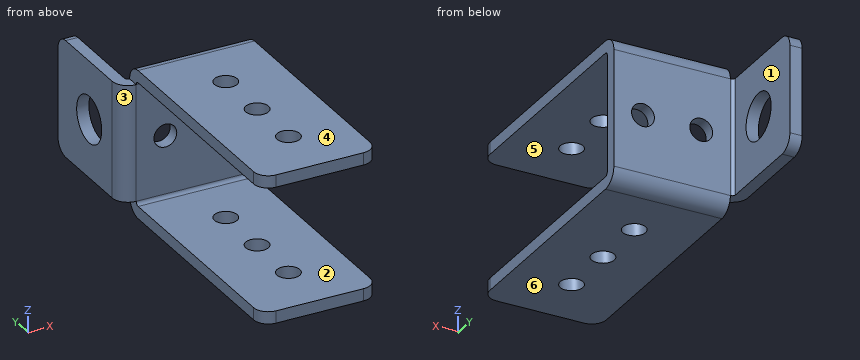
```python
from build123d import *

# Parameters (mm, degrees)
BASE_FLANGE1_START = -12.7
BASE_FLANGE1_DEPTH = 25.4
EDGE_FLANGE1_DEPTH = 25.4
SKETCH9_R          = 5.08
CUT_EXTRUDE1_DEPTH = 86.828419099
SKETCH10_R         = 2.4892
CUT_EXTRUDE2_DEPTH = 85.303992818
CUT_EXTRUDE3_REACH = 65.202
SKETCH11_R         = 2.4892
FILLET1_R          = 3.175


# Read off the part's stored shape, not the designer's step: Base-Flange1
# Sheet-metal steps are written as plain solids
with BuildPart() as part:
    # Base-Flange1 outline → Base-Flange1 (new body)
    with BuildSketch(Plane(origin=(0, 0, 0), x_dir=(0, 0, -1), z_dir=(1, 0, 0)).offset(BASE_FLANGE1_START)):
        with BuildLine():
            Line((26.924, 50.038), (26.924, 0))
            Line((26.924, 0), (29.591, 0))
            Line((29.591, 0), (29.591, 50.038))
            ThreePointArc((29.591, 50.038), (28.586669153, 52.462669153), (26.162, 53.467))
            Line((26.162, 53.467), (0.762, 53.467))
            ThreePointArc((0.762, 53.467), (-1.662669153, 52.462669153), (-2.667, 50.038))
            Line((-2.667, 50.038), (-2.667, 0))
            Line((-2.667, 0), (0, 0))
            Line((0, 0), (0, 50.038))
            ThreePointArc((0, 50.038), (0.223184633, 50.576815367), (0.762, 50.8))
            Line((0.762, 50.8), (26.162, 50.8))
            ThreePointArc((26.162, 50.8), (26.700815367, 50.576815367), (26.924, 50.038))
        make_face()
    extrude(amount=BASE_FLANGE1_DEPTH)

    # Edge-Flange1 section (across the edge) → Edge-Flange1 (add)
    with BuildSketch(Plane(origin=(-13.462, 53.467, -26.162), x_dir=(1, 0, 0), z_dir=(0, 0, 1))):
        with BuildLine():
            Line((-2.667, 0.762), (-2.667, 22.733))
            Line((-2.667, 22.733), (0, 22.733))
            Line((0, 22.733), (0, 0.762))
            ThreePointArc((0, 0.762), (0.223184633, 0.223184633), (0.762, 0))
            Line((0.762, 0), (0.762, -2.667))
            ThreePointArc((0.762, -2.667), (-1.662669153, -1.662669153), (-2.667, 0.762))
        make_face()
    extrude(amount=EDGE_FLANGE1_DEPTH)

    # Sketch9 → Cut-Extrude1 (cut, through all)
    with BuildSketch(Plane(origin=(-13.462, 0, 0), x_dir=(0, 0, -1), z_dir=(1, 0, 0))):
        with Locations(Location((13.462, 63.5, 0), (0, 0, 90))):
            Circle(SKETCH9_R)
    extrude(amount=-CUT_EXTRUDE1_DEPTH, mode=Mode.SUBTRACT)

    # Sketch10 → Cut-Extrude2 (cut, through all)
    with BuildSketch(Plane.XY.offset(2.667)):
        with Locations((0, 12.7)):
            Circle(SKETCH10_R)
        with Locations((0, 25.4)):
            Circle(SKETCH10_R)
        with Locations((0, 38.1)):
            Circle(SKETCH10_R)
    extrude(amount=-CUT_EXTRUDE2_DEPTH, mode=Mode.SUBTRACT)

    # Sketch11 → Cut-Extrude3 (cut, up to next)
    with BuildSketch(Plane(origin=(0, 53.467, 0), x_dir=(1, 0, 0), z_dir=(0, 1, 0)), mode=Mode.PRIVATE) as cut_extrude3_sk1:
        with Locations(Location((-6.35, 13.462, 0), (0, 0, 270))):
            Circle(SKETCH11_R)
    cut_extrude3_tool1 = extrude(cut_extrude3_sk1.sketch, amount=-CUT_EXTRUDE3_REACH, mode=Mode.PRIVATE) & part.part
    # Sketch11 → Cut-Extrude3 (cut, up to next)
    with BuildSketch(Plane(origin=(0, 53.467, 0), x_dir=(1, 0, 0), z_dir=(0, 1, 0)), mode=Mode.PRIVATE) as cut_extrude3_sk2:
        with Locations(Location((6.35, 13.462, 0), (0, 0, 270))):
            Circle(SKETCH11_R)
    cut_extrude3_tool2 = extrude(cut_extrude3_sk2.sketch, amount=-CUT_EXTRUDE3_REACH, mode=Mode.PRIVATE) & part.part
    add(cut_extrude3_tool1.solids().sort_by_distance((-6.35, 53.467, -13.462))[0], mode=Mode.SUBTRACT)
    add(cut_extrude3_tool2.solids().sort_by_distance((6.35, 53.467, -13.462))[0], mode=Mode.SUBTRACT)

    # Fillet1
    fillet1_edges = [part.edges().sort_by_distance(p)[0] for p in [
        (-12.7, 0, 1.3335),
        (-12.7, 0, -28.2575),
        (12.7, 0, 1.3335),
        (-14.7955, 76.2, -26.162),
        (-14.7955, 76.2, -0.762),
        (12.7, 0, -28.2575),
    ]]
    fillet(fillet1_edges, radius=FILLET1_R)


solid = part.part
```
Input: part model. Units: mm. Frame: model coordinates. Face numbers are marked on the shaded views. A direction names the side the tool comes from. Round coordinates to 2 decimals unless told otherwise and drop trailing zeros. Loops run counter-clockwise (first coordinate to the right, second up) from the corner with the lowest first, then second, coordinate; pieces in that order, holes last. Notation, with made-up numbers: (89.25, 45) -> (143.25, 45) arc R18 ccw to (143.25, 61) -> close; hole circle Ø6 at (58, 84). An arc over 180 degrees is marked (long way). Write each question's results on one line, items separated by ' | '.
1. Ray query, line 1 (Z direction, x = -15.55, y = 63.5); line 2 (Z direction, x = -10.25, y = 17.5); line 3 (Y direction, x = 0, z = 1.6). Return the intervals inside material, ascending. Write a range as from..to.
Geometry results:
line 1: -26.16..-18.54, -8.38..-0.76 | line 2: -29.59..-26.92, 0..2.67 | line 3: 0..10.21, 15.19..22.91, 27.89..35.61, 40.59..52.52
2. Section B-B (y = 25.4). Return loops of the section in (x, z), and give its area (3 significant figures).
Geometry results:
outline: (-12.7, -29.59) -> (-2.49, -29.59) -> (-2.49, -26.92) -> (-12.7, -26.92) -> close; (-12.7, 0) -> (-2.49, 0) -> (-2.49, 2.67) -> (-12.7, 2.67) -> close; (2.49, -29.59) -> (12.7, -29.59) -> (12.7, -26.92) -> (2.49, -26.92) -> close; (2.49, 0) -> (12.7, 0) -> (12.7, 2.67) -> (2.49, 2.67) -> close | area: 109 mm2
3. Set-up query: the marked faces 1, 2 and 3. Return all of +Z, -Z, +X, -X, +Y, -Y with unobstructed straight access to the full face (end or side cutting, diameter ignored); none if empty.
Geometry results:
face 1: +Z, -Z, +X, +Y | face 2: +X, -X, -Y | face 3: +Z, -Z, -X, -Y
4. First-contact query: P1, Ø4.5, axis at x = 0, y = 38.1, coming from the -Z side; P2, Ø6.5, axis at x = -6.35, z = -13.462, coming from the -Y side; P3, Ø2, axis at x = 9.5, z = -4, coming from the +Y side; P4, Ø1.5, axis at y = 51.5, z = -5.5, coming from the -X side. Flat tips, straight axial feed; report the tip coordinate or a pass-through.
Geometry results:
P1: through | P2: y = 50.8 | P3: y = 53.47 | P4: x = -15.5
5. Section C-C (z = -12). Return loops of the section in (x, y).
Geometry results:
outline: (-16.13, 54.23) arc R3.43 ccw to (-12.7, 50.8) -> (-8.36, 50.8) -> (-8.36, 53.47) -> (-12.7, 53.47) arc R0.76 cw to (-13.46, 54.23) -> (-13.46, 58.63) -> (-16.13, 58.63) -> close; (-16.13, 68.37) -> (-13.46, 68.37) -> (-13.46, 76.2) -> (-16.13, 76.2) -> close; (-4.34, 50.8) -> (4.34, 50.8) -> (4.34, 53.47) -> (-4.34, 53.47) -> close; (8.36, 50.8) -> (12.7, 50.8) -> (12.7, 53.47) -> (8.36, 53.47) -> close
6. Mould query, pull axis Z, two halves, no side actions, for the marked faces 4, 5 and 6. Classes: +Z half, -Z half, draft (parallel to the pull), parting line (faces both ways), or undercut.
Geometry results:
face 4: +Z half | face 5: undercut | face 6: -Z half
7. Section A-A (x = 6.35). Return loops of the section in (y, z).
Geometry results:
outline: (0, -29.59) -> (50.04, -29.59) arc R3.43 ccw to (53.47, -26.16) -> (53.47, -15.95) -> (50.8, -15.95) -> (50.8, -26.16) arc R0.76 cw to (50.04, -26.92) -> (0, -26.92) -> close; (0, 0) -> (50.04, 0) arc R0.76 cw to (50.8, -0.76) -> (50.8, -10.97) -> (53.47, -10.97) -> (53.47, -0.76) arc R3.43 ccw to (50.04, 2.67) -> (0, 2.67) -> close
8. Section D-D (y = 34.5). Return loops of the section in (x, z).
Geometry results:
outline: (-12.7, -29.59) -> (12.7, -29.59) -> (12.7, -26.92) -> (-12.7, -26.92) -> close; (-12.7, 0) -> (12.7, 0) -> (12.7, 2.67) -> (-12.7, 2.67) -> close
